```python
from build123d import *

# Parameters (mm, degrees)
SKETCH1_R           = 24.60625
BOSS_EXTRUDE1_DEPTH = 5.55625
SKETCH2_R           = 14.2875
BOSS_EXTRUDE2_DEPTH = 0.79375
SKETCH3_R           = 11.1125
CUT_EXTRUDE1_DEPTH  = 36.373119429
FILLET1_R           = 1


with BuildPart() as part:
    # Sketch1 → Boss-Extrude1 (new body)
    with BuildSketch(Plane(origin=(0, 0, 0), x_dir=(1, 0, 0), z_dir=(0, 1, 0))):
        with Locations(Location((0, 0, 0), (0, 0, 270))):
            Circle(SKETCH1_R)
    extrude(amount=BOSS_EXTRUDE1_DEPTH)

    # Sketch2 → Boss-Extrude2 (add)
    with BuildSketch(Plane(origin=(0, 5.55625, 0), x_dir=(1, 0, 0), z_dir=(0, 1, 0))):
        with Locations(Location((0, 0, 0), (0, 0, 270))):
            Circle(SKETCH2_R)
    extrude(amount=BOSS_EXTRUDE2_DEPTH)

    # Sketch3 → Cut-Extrude1 (cut, through all)
    with BuildSketch(Plane(origin=(0, 6.35, 0), x_dir=(1, 0, 0), z_dir=(0, 1, 0))):
        with Locations(Location((0, 0, 0), (0, 0, 270))):
            Circle(SKETCH3_R)
    extrude(amount=-CUT_EXTRUDE1_DEPTH, mode=Mode.SUBTRACT)

    # Fillet1
    # the kernel refuses this fillet: 1 mm, written as the material it adds along each edge
    with BuildSketch(Plane(origin=(0, 5.55625, 0), x_dir=(0, 0, 1), z_dir=(-1, 0, 0))) as fillet1_piece_1:
        with BuildLine():
            CenterArc((15.265999329, 1), FILLET1_R, 191.902682649, 78.097317351)
            Line((14.2875, 0.79375), (14.267930013, 0.789625))
            ThreePointArc((14.267930013, 0.789625), (14.2675, 0.396875), (14.2675, 0))
            Line((14.2675, 0), (14.2875, -0.02))
            Line((14.2875, -0.02), (15.265999329, -0.02))
            Line((15.265999329, -0.02), (15.265999329, 0))
        make_face()
    revolve(axis=Axis((0, 5.55625, 0), (0, 1, 0)))


solid = part.part
```
Geometry check sheet. Reference: the model listing, model coordinates, mm. A direction names the side the tool comes from. Coordinates: 2 decimals unless noted, no trailing zeros. Write each loop counter-clockwise with the first axis right and the second up, starting at its lowest first coordinate (ties: lowest second). Pieces come first, ordered by that corner, then holes. Notation, with made-up numbers: M -14.5,37 L -2.5,37 A19 cw -2.5,50 Z; hole C 0.5,-3 d10. An arc over 180 degrees is marked long. Answer as a JSON object with one key per item and string values.
1. Section check C-C, the plane y = 1.5. Enter the section's corners in (x, z) (1 decimal).
Answers below:
{"outline": "C 0,0 d49.2; hole C 0,0 d22.2"}
2. Scan lines: L1, parallel to X at y = 4.75, z = 0; L2, parallel to X at y = 4.5, z = -3.5; L3, parallel to Y at x = 21.5, z = 10. Record each from-to range of solid material in increasing order.
Answers below:
{"L1": "x = -24.61 to -11.11, 11.11 to 24.61", "L2": "x = -24.36 to -10.55, 10.55 to 24.36", "L3": "y = 0 to 5.56"}
3. Section check A-A, the plane z = 0. Enter the section's corners in (x, y), plus the area to 3 significant figures.
Answers below:
{"outline": "M -24.61,0 L -11.11,0 L -11.11,6.35 L -14.29,6.35 A1 cw -15.27,5.56 L -24.61,5.56 Z; M 11.11,0 L 24.61,0 L 24.61,5.56 L 15.27,5.56 A1 cw 14.29,6.35 L 11.11,6.35 Z", "area": "155 mm²"}
4. Go/stop test with flat-tipped pins: pin 1 Ø1.5 at (x, y) = (-15, 1) entering from +Z; pin 2 Ø1.5 at (y, z) = (1, -16.5) entering from +X; pin 3 Ø3 at (x, y) = (-7.5, 4.5) entering from +Z. Record where each tip stops, or that it passes through.
Answers below:
{"pin 1": "stops at z = 20.06", "pin 2": "stops at x = 18.91", "pin 3": "stops at z = 23.86"}
5. Section check D-D, the plane x = -21.5. Enter the section's corners in (y, z).
Answers below:
{"outline": "M 0,-11.97 L 5.56,-11.97 L 5.56,11.97 L 0,11.97 Z"}
6. Section check B-B, the plane x = 0. Enter the section's corners in (y, z).
Answers below:
{"outline": "M 0,-24.61 L 5.56,-24.61 L 5.56,-15.27 A1 cw 6.35,-14.29 L 6.35,-11.11 L 0,-11.11 Z; M 0,11.11 L 6.35,11.11 L 6.35,14.29 A1 cw 5.56,15.27 L 5.56,24.61 L 0,24.61 Z"}
7. Draft check along Z on faces 1 (the cylindrical face through (9.37, 3.219, 5.974)), 2 (the cylindrical face through (24.397, 2.739, -3.203)), 3 (the flat face through (-7, 6.35, -9)). Enter one of: released by +Z, released by -Z, zero draft, split by the parting line, or undercut.
Answers below:
{"face 1": "undercut", "face 2": "split by the parting line", "face 3": "zero draft"}
8. Tool access check on faces 4 (the flat face through (-5, 0, 11)), 5 (the flat face through (-11, 5.556, -11)). Record the directions out of +Z, -Z, +X, -X, +Y, -Y that give a thin tool (end or side, any length) a straight path to the whole face; none if there is none.
Answers below:
{"face 4": "+Z, -Z, +X, -X, -Y", "face 5": "+Y"}
